Can you work these out from the drawing? Everything is in mm from the part's minimum corner. A direction names the side the tool comes from. Give positions to 0.01 mm unless a question says otherwise; leave off trailing zeros. Loops run counter-clockwise (first coordinate to the right, second up) from the corner with the lowest first, then second, coordinate; pieces in that order, holes last.
Q1. If we section it at C-C (y = 3.5): Please give me the cut outline in (x, z).
Q2. For the marked faces 1 and 2, which set-ups out of +Z, -Z, +X, -X, +Y, -Y let a thin tool reach every point of the face, with its end or its side?
Q3. Will these pins go through, and if not, where does the flat tip stop? P1, Ø0.8, axis at x = 2, y = 7, coming from the -Z side; P2, Ø0.8, axis at x = 0.5, y = 10, coming from the +Z side; P3, Ø0.8, axis at x = 2, z = 17.5, coming from the +Y side.
Q4. If we section it at D-D (y = 16.25): Please give me the cut outline in (x, z).
Q5. If we section it at A-A (z = 18): Please give me the cut outline in (x, y).
Q6. If we section it at B-B (x = 33): Please give me the cut outline in (y, z), plus the area to 3 significant figures.
Q7. I need wall thicknesses on line 1 (X direction, y = 1.75, z = 4.25); line 2 (Z direction, x = 22, y = 15.5); line 3 (Z direction, x = 38.5, y = 15.75). Which ranges of each line are inside material? Lowest first, please.
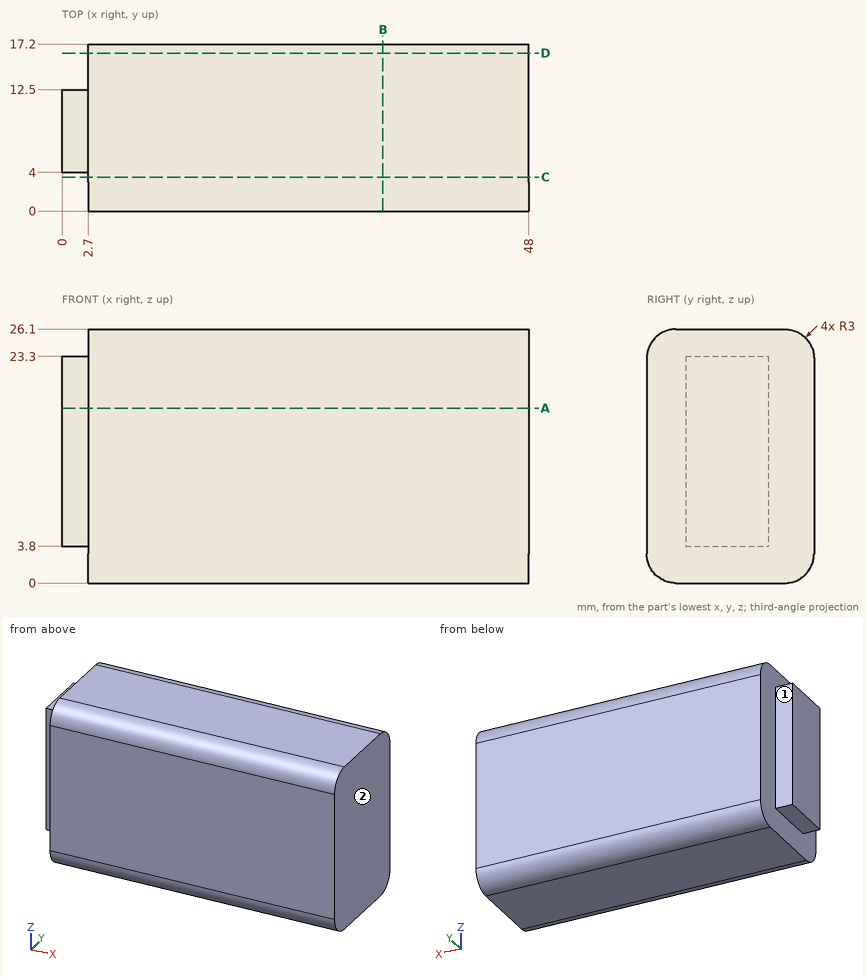
Check sheet entries:
1. outline: (2.7, 0) - (48, 0) - (48, 26.1) - (2.7, 26.1) - close
2. face 1: +Z, -Z, -X, +Y
2. face 2: +Z, -Z, +X, +Y, -Y
3. P1: stops at z = 3.8
3. P2: stops at z = 23.3
3. P3: stops at y = 12.5
4. outline: (2.7, 0.81) - (48, 0.81) - (48, 25.29) - (2.7, 25.29) - close
5. outline: (0, 4) - (2.7, 4) - (2.7, 0) - (48, 0) - (48, 17.2) - (2.7, 17.2) - (2.7, 12.5) - (0, 12.5) - close
6. outline: (0, 3) arc R3 ccw to (3, 0) - (14.2, 0) arc R3 ccw to (17.2, 3) - (17.2, 23.1) arc R3 ccw to (14.2, 26.1) - (3, 26.1) arc R3 ccw to (0, 23.1) - close
6. area: 441 mm2
7. line 1: x = 2.7 to 48
7. line 2: z = 0.3 to 25.8
7. line 3: z = 0.43 to 25.67
